from build123d import *

# Parameters (mm, degrees)
SKETCH1_R           = 25
SKETCH1_R_2         = 23.75
BOSS_EXTRUDE1_DEPTH = 2.75
SKETCH2_R           = 23.75
BOSS_EXTRUDE2_DEPTH = 0.5


with BuildPart() as part:
    # Sketch1 → Boss-Extrude1 (new body, symmetric)
    with BuildSketch(Plane.XY):
        Circle(SKETCH1_R)
        Circle(SKETCH1_R_2, mode=Mode.SUBTRACT)
    extrude(amount=BOSS_EXTRUDE1_DEPTH, both=True)

    # Sketch2 → Boss-Extrude2 (add, symmetric)
    with BuildSketch(Plane.XY):
        Circle(SKETCH2_R)
    extrude(amount=BOSS_EXTRUDE2_DEPTH, both=True)


solid = part.part
The model under review builds one solid part; all positions refer to its coordinate system, in mm. A direction names the side the tool comes from. Coordinates: 2 decimals unless noted, no trailing zeros. Order: outer loops, then holes, each group sorted by start corner. A loop starts at its lowest first (then second) coordinate and runs counter-clockwise, first axis right, second up. Notation, with made-up numbers: (83, 77) -> (117, 77) arc R22 ccw to (117, 116) -> close; hole circle Ø1 at (-11.75, 29.25). An arc over 180 degrees is marked (long way). Answer in a Markdown table with one row per item.
(1) Consider section C-C (y = 8). Write out the cut boundary in (x, z).
Answers:
| item | result |
|---|---|
| outline | (-23.69, -2.75) -> (-22.36, -2.75) -> (-22.36, -0.5) -> (22.36, -0.5) -> (22.36, -2.75) -> (23.69, -2.75) -> (23.69, 2.75) -> (22.36, 2.75) -> (22.36, 0.5) -> (-22.36, 0.5) -> (-22.36, 2.75) -> (-23.69, 2.75) -> close |
(2) Machinability: for faces 4 (the cylindrical face through (-5.149, -23.185, 1.609)), 5 (the flat face through (0, 0, -0.5)), 6 (the flat face through (22.1, -9.1, 2.75)), which of the approach directions +Z, -Z, +X, -X, +Y, -Y give a long, thin tool a straight path to every point of the face, cutting with its end or side? Answer none if there is none.
Answers:
| item | result |
|---|---|
| face 4 | +Z |
| face 5 | -Z |
| face 6 | +Z, +X, -X, +Y, -Y |
(3) The part is to be moulded in two halves that separate along X. For faces 1 (the cylindrical face through (23.846, 7.509, 0.038)), 2 (the flat face through (0, 0, 0.5)), 3 (the flat face through (22.1, -9.1, -2.75)), say which applies: +X half, -X half, draft (parallel to the pull), parting line (faces both ways), or undercut.
Answers:
| item | result |
|---|---|
| face 1 | parting line |
| face 2 | undercut |
| face 3 | draft |
(4) Consider section B-B (x = 0). Write out the cut boundary in (y, z), plus the area to 4 significant figures.
Answers:
| item | result |
|---|---|
| outline | (-25, -2.75) -> (-23.75, -2.75) -> (-23.75, -0.5) -> (23.75, -0.5) -> (23.75, -2.75) -> (25, -2.75) -> (25, 2.75) -> (23.75, 2.75) -> (23.75, 0.5) -> (-23.75, 0.5) -> (-23.75, 2.75) -> (-25, 2.75) -> close |
| area | 61.25 mm² |
(5) Wall thickness on line 1 along Z through (x, y) = (-8.5, 9.5); line 2 along Y through (x, z) = (-3, 0.6); line 3 along X through (y, z) = (20.5, -2.4): over which ranges is each line inside the solid? List them lowest first.
Answers:
| item | result |
|---|---|
| line 1 | -0.5 to 0.5 |
| line 2 | -24.82 to -23.56, 23.56 to 24.82 |
| line 3 | -14.31 to -11.99, 11.99 to 14.31 |
(6) Insertion check: pin 1 (2 mm diameter, centred on x = -1.5, z = 0, fed in from -Y) (3 decimals); pin 2 (2 mm diameter, centred on x = 2, z = 2, fed in from +Y); pin 3 (1.5 mm diameter, centred on y = 13.5, z = -1, fed in from -X). Each pin has a flat end and moves straight along its axis. Give the tip position at first contact, or say it passes through.
Answers:
| item | result |
|---|---|
| pin 1 | y = -24.995 |
| pin 2 | y = 24.98 |
| pin 3 | x = -21.5 |
(7) Consider section A-A (z = -2.1). Write out the cut boundary in (x, y).
Answers:
| item | result |
|---|---|
| outline | circle Ø50 at (0, 0); hole circle Ø47.5 at (0, 0) |
